Verification items for the finished model (mm, model axes). Face numbers are marked on the shaded views. A direction names the side the tool comes from. Coordinates: 2 decimals unless noted, no trailing zeros. Write each loop counter-clockwise with the first axis right and the second up, starting at its lowest first coordinate (ties: lowest second). Pieces come first, ordered by that corner, then holes. Notation, with made-up numbers: (-5.75, 12.25) -> (48.25, 12.25) arc R21 ccw to (48.25, 38.25) -> close; hole circle Ø2 at (23, 76). An arc over 180 degrees is marked (long way). Write item = value, one per line. Start each with the question number.
(1) Material ranges on probe 1 along X at (y, z) = (-2.1, 0.5); probe 2 along Z at (x, y) = (-15.5, 0), recorded low to high. Write a range as [from, to].
(2) Mould release check, pull along Y, two halves, no side actions. Record for the marked faces 3 and 4: released by +Y, released by -Y, zero draft, split by the parting line, or undercut.
(3) Gauge pin test, flat ends, axial feed: pin 1 Ø2 at (y, z) = (0, 0) entering from +X; pin 2 Ø1.5 at (x, z) = (-5.5, 0.5) entering from -Y. Record the tip position at first contact, or that the pin passes through.
(4) Section check D-D (x = -15.5). Record the cut outline in (y, z), plus the area to 3 significant figures.
(5) Set-up check for the marked faces 1 and 2: record each of +Z, -Z, +X, -X, +Y, -Y from which the full face is reachable in a straight line by a thin tool's end or side.
(6) Section check C-C (x = -22.75). Record the cut outline in (y, z) (3 decimals).
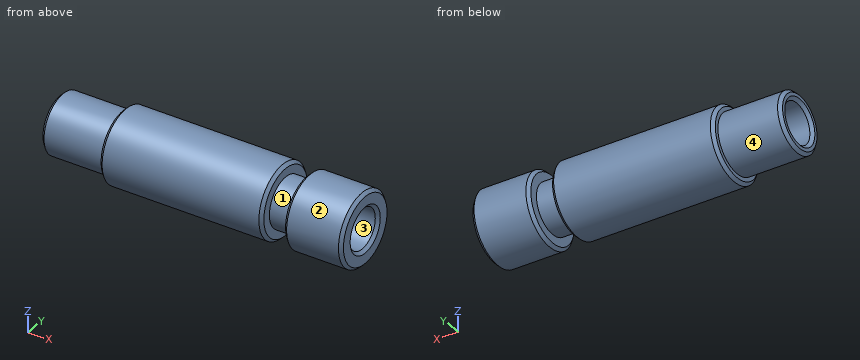
Autodesk Inventor part; units mm, degrees
ref_plane "YZ Plane" through (0, 0, 0) normal (1, 0, 0) x (0, 1, 0)
ref_plane "XZ Plane" through (0, 0, 0) normal (0, 1, 0) x (-1, 0, 0)
ref_plane "XY Plane" through (0, 0, 0) normal (0, 0, 1) x (1, 0, 0)
sketch "Esquisse1" plane through (0, 0, 0) normal (0, 0, 1) x (1, 0, 0)
  line L0 (0, 1.65) -> (0, 3)
  line L1 (0, 3) -> (-4.8, 3)
  line L2 (-4.8, 3) -> (-4.8, 2.05)
  line L3 (-4.8, 2.05) -> (-6.6, 2.05)
  line L4 (-6.6, 2.05) -> (-6.6, 3)
  line L5 (-6.6, 3) -> (-20.1, 3)
  line L6 (-20.1, 3) -> (-20.1, 2.425)
  line L7 (-20.1, 2.425) -> (-25.3, 2.425)
  line L8 (-25.3, 2.425) -> (-25.3, 1.65)
  line L9 (-25.3, 1.65) -> (0, 1.65)
  line L10 (0, 0) -> (-19.9979, 0)
  dimension "d0" = 6
  dimension "d1" = 3.3
  dimension "d2" = 4.1
  dimension "d3" = 4.8
  dimension "d4" = 13.5
  dimension "d5" = 1.8
  dimension "d6" = 4.85
  dimension "d7" = 25.3
revolve "Révolution1" add sketch "Esquisse1" angle 360 about axis through (0, 0, 0) along (-1, 0, 0)
chamfer "Chanfrein1" distance 0.25 angle 45 7 edges at (0, -1.65, 0) (0, -3, 0) (-25.3, -2.425, 0) (-25.3, -1.65, 0) (-4.8, -3, 0) (-6.6, -3, 0) (-20.1, -3, 0)
thread "Filetage1"
thread "Filetage2"
properties part number "Vis de raccord" material "Acier"
Response:
q1.probe_1 = [-25.3, -6.6], [-4.8, 0]
q1.probe_2 = [-3, -1.65], [1.65, 3]
q2.face_3 = undercut
q2.face_4 = split by the parting line
q3.pin_1 = through
q3.pin_2 = -2.76
q4.outline = circle Ø6 at (0, 0); hole circle Ø3.3 at (0, 0)
q4.area = 19.7 mm2
q5.face_1 = none
q5.face_2 = +X, -X
q6.outline = circle Ø4.85 at (0, 0); hole circle Ø3.3 at (0, 0)
